Design review of the part built by this model. Coordinates are the model's own, in mm. A direction names the side the tool comes from. Give positions to 0.01 mm unless a question says otherwise; leave off trailing zeros. Write each loop counter-clockwise with the first axis right and the second up, starting at its lowest first coordinate (ties: lowest second). Pieces come first, ordered by that corner, then holes.
```python
from build123d import *

# Parameters (mm, degrees)
SKETCH1_R           = 1.6
BOSS_EXTRUDE1_DEPTH = 1.6


with BuildPart() as part:
    # Sketch1 → Boss-Extrude1 (new body)
    with BuildSketch(Plane.XY):
        with BuildLine():
            Line((-58.5, -3), (-55.91958512, -3))
            ThreePointArc((-55.91958512, -3), (-39.597979746, -39.597979746), (-3, -55.91958512))
            Line((-3, -55.91958512), (-3, -58.5))
            ThreePointArc((-3, -58.5), (0, -61.5), (3, -58.5))
            Line((3, -58.5), (3, -55.91958512))
            ThreePointArc((3, -55.91958512), (39.597979746, -39.597979746), (55.91958512, -3))
            Line((55.91958512, -3), (58.5, -3))
            ThreePointArc((58.5, -3), (61.5, 0), (58.5, 3))
            Line((58.5, 3), (55.91958512, 3))
            ThreePointArc((55.91958512, 3), (39.597979746, 39.597979746), (3, 55.91958512))
            Line((3, 55.91958512), (3, 58.5))
            ThreePointArc((3, 58.5), (0, 61.5), (-3, 58.5))
            Line((-3, 58.5), (-3, 55.91958512))
            ThreePointArc((-3, 55.91958512), (-39.597979746, 39.597979746), (-55.91958512, 3))
            Line((-55.91958512, 3), (-58.5, 3))
            ThreePointArc((-58.5, 3), (-61.5, 0), (-58.5, -3))
        make_face()
        with Locations((-41, 0)):
            Circle(SKETCH1_R, mode=Mode.SUBTRACT)
        with Locations((0, -41)):
            Circle(SKETCH1_R, mode=Mode.SUBTRACT)
        with Locations((41, 0)):
            Circle(SKETCH1_R, mode=Mode.SUBTRACT)
        with Locations((0, 41)):
            Circle(SKETCH1_R, mode=Mode.SUBTRACT)
        with Locations((-58.5, 0)):
            Circle(SKETCH1_R, mode=Mode.SUBTRACT)
        with Locations((0, 58.5)):
            Circle(SKETCH1_R, mode=Mode.SUBTRACT)
        with Locations((58.5, 0)):
            Circle(SKETCH1_R, mode=Mode.SUBTRACT)
        with Locations((0, -58.5)):
            Circle(SKETCH1_R, mode=Mode.SUBTRACT)
        with BuildLine():
            ThreePointArc((44.899888641, 3), (31.819805153, 31.819805153), (3, 44.899888641))
            Line((3, 44.899888641), (3, 41))
            ThreePointArc((3, 41), (0, 38), (-3, 41))
            Line((-3, 41), (-3, 44.899888641))
            ThreePointArc((-3, 44.899888641), (-31.819805153, 31.819805153), (-44.899888641, 3))
            Line((-44.899888641, 3), (-41, 3))
            ThreePointArc((-41, 3), (-38, 0), (-41, -3))
            Line((-41, -3), (-44.899888641, -3))
            ThreePointArc((-44.899888641, -3), (-31.819805153, -31.819805153), (-3, -44.899888641))
            Line((-3, -44.899888641), (-3, -41))
            ThreePointArc((-3, -41), (0, -38), (3, -41))
            Line((3, -41), (3, -44.899888641))
            ThreePointArc((3, -44.899888641), (31.819805153, -31.819805153), (44.899888641, -3))
            Line((44.899888641, -3), (41, -3))
            ThreePointArc((41, -3), (38, 0), (41, 3))
            Line((41, 3), (44.899888641, 3))
        make_face(mode=Mode.SUBTRACT)
    extrude(amount=BOSS_EXTRUDE1_DEPTH)


solid = part.part
```
(1) Clearance check with flat-ended pins moving along their axes: P1, Ø0.5, axis at x = -43, z = 0.5, coming from the -Y side; P2, Ø0.5, axis at y = 43, z = 1, coming from the +X side; P3, Ø0.8, axis at x = -43, z = 1, coming from the +Y side. State where each tip first meets the part, or that it passes through.
Resolved:
P1: stops at y = -36.17
P2: stops at x = 36.17
P3: stops at y = 36.35
(2) Consider section C-C, the plane y = 29. Give the boundary of the cut face in (x, z), then the cut area to 3 significant figures.
Resolved:
outline: (-47.91, 0) - (-34.41, 0) - (-34.41, 1.6) - (-47.91, 1.6) - close; (34.41, 0) - (47.91, 0) - (47.91, 1.6) - (34.41, 1.6) - close
area: 43.2 mm2
(3) Tool access review of faces 4 (the face through (-32, 32, 0)), 5 (the face through (38, 0, 1)): name each direction out of +Z, -Z, +X, -X, +Y, -Y from which nothing blocks a thin tool from reaching the whole face with its end or side.
Resolved:
face 4: -Z, +X, -X, +Y, -Y
face 5: +Z, -Z
(4) To check wall thickness, follow L1, parallel to Y at x = 0, z = 0.6; L2, parallel to X at y = 40.5, z = 1; L3, parallel to X at y = -1, z = 0.4. State the ranges of each line that lie inside material, in increasing order.
Resolved:
L1: y = -61.5 to -60.1, -56.9 to -42.6, -39.4 to -38, 38 to 39.4, 42.6 to 56.9, 60.1 to 61.5
L2: x = -38.67 to -19.62, -2.96 to -1.52, 1.52 to 2.96, 19.62 to 38.67
L3: x = -61.33 to -59.75, -57.25 to -42.25, -39.75 to -38.17, 38.17 to 39.75, 42.25 to 57.25, 59.75 to 61.33
(5) Consider section B-B, the plane x = 18. Give the boundary of the cut face in (y, z).
Resolved:
outline: (-53.03, 0) - (-41.24, 0) - (-41.24, 1.6) - (-53.03, 1.6) - close; (41.24, 0) - (53.03, 0) - (53.03, 1.6) - (41.24, 1.6) - close
(6) Consider section A-A, the plane x = 0. Give the boundary of the cut face in (y, z), then the cut area to 3 significant figures.
Resolved:
outline: (-61.5, 0) - (-60.1, 0) - (-60.1, 1.6) - (-61.5, 1.6) - close; (-56.9, 0) - (-42.6, 0) - (-42.6, 1.6) - (-56.9, 1.6) - close; (-39.4, 0) - (-38, 0) - (-38, 1.6) - (-39.4, 1.6) - close; (38, 0) - (39.4, 0) - (39.4, 1.6) - (38, 1.6) - close; (42.6, 0) - (56.9, 0) - (56.9, 1.6) - (42.6, 1.6) - close; (60.1, 0) - (61.5, 0) - (61.5, 1.6) - (60.1, 1.6) - close
area: 54.7 mm2
(7) Mouldability with a two-part tool opening along Y and no side actions: class faces 1 (the face through (0, 38, 1)), 2 (the face through (61.5, -0.1, 0.8)), 3 (the face through (-32, 32, 1.6)) as pulls with the +Y half, pulls with the -Y half, needs draft (parallel to the pull), parting line crosses it, or undercut.
Resolved:
face 1: undercut
face 2: parting line crosses it
face 3: needs draft
(8) Consider section D-D, the plane z = 1.35. Give the number of separate pieces and of enclosed holes in the cut face, then the cut area to 3 significant figures.
Resolved:
separate pieces: 1
enclosed holes: 9
area: 3,690 mm2
